Autodesk Inventor part; units mm, degrees
ref_plane "YZ Plane" through (0, 0, 0) normal (1, 0, 0) x (0, 1, 0)
ref_plane "XZ Plane" through (0, 0, 0) normal (0, 1, 0) x (-1, 0, 0)
ref_plane "XY Plane" through (0, 0, 0) normal (0, 0, 1) x (1, 0, 0)
sketch "スケッチ1" plane through (0, 0, 0) normal (0, 0, 1) x (1, 0, 0)
  line L0 (0, 0) -> (-57.5, 0)
  line L1 (-57.5, 0) -> (-57.5, 28)
  line L2 (-57.5, 28) -> (0, 28)
  line L3 (0, 28) -> (0, 0)
  line L4 (0, 14) -> (-110.5, 14)
  circle A0 centre (-110.5, 14) radius 53
  circle A1 centre (-110.5, 14) radius 23.5
  line L5 (0, 28) -> (-108.4685, 37.412)
  line L6 (0, 0) -> (-108.4685, -9.412)
  point P0 (-108.4685, -9.412)
  dimension "d3" = 47
  dimension "d0" = 28
  dimension "d1" = 57.5
  dimension "d2" = 106
extrude "押し出し1" add sketch "スケッチ1" along normal blind 3 contours L6 A0 L1 L0 | L0 L1 L4 L3 | L4 L1 L2 L3 | L6 A1 L4 A0 | A0 L5 L2 L1 | L4 A1 L5 A0 | A1
sketch "スケッチ2" plane through (0, 0, 3) normal (0, 0, 1) x (1, 0, 0)
  line L0 (0, 28) -> (-108.4685, 37.412)
  line L1 (0, 28) -> (-47.5, 28)
  line L2 (-47.5, 28) -> (-47.5, 0)
  line L3 (-47.5, 0) -> (0, 0)
  line L4 (0, 0) -> (0, 28)
  line L5 (-5, 28) -> (-5, 0)
  line L6 (-35, 28) -> (-35, 0)
  line L7 (0, 14) -> (-47.5, 14)
  point P0 (-35, 24)
  point P1 (-5, 24)
  point P2 (-35, 4)
  point P3 (-5, 4)
  dimension "d6" = 28
  dimension "d7" = 47.5
  dimension "d8" = 5
  dimension "d9" = 30
  dimension "d10" = 10
  dimension "d11" = 10
hole "穴1" at (-35, 24, 3) at (-5, 24, 3) at (-35, 4, 3) at (-5, 4, 3) direction (0, 0, -1) diameter 3.1 end through all
sketch "スケッチ3" plane through (0, 0, 3) normal (0, 0, 1) x (1, 0, 0)
  arc A0 (-108.4685, 37.412) -> (-108.4685, -9.412) centre (-110.5, 14) ccw
  circle A1 centre (-110.5, 14) radius 15.18
  circle A2 centre (-110.5, 14) radius 6
  line L0 (-110.5, 14) -> (-118.09, 27.1463)
  line L1 (-123.6463, 21.59) -> (-110.5, 14)
  line L2 (-110.5, 14) -> (-102.91, 27.1463)
  line L3 (-110.5, 14) -> (-110.5, 29.18)
  point P0 (0, 0)
  point P1 (-123.6463, 6.41)
  point P2 (-110.5, -1.18)
  point P3 (-97.3537, 6.41)
  point P4 (-97.3537, 21.59)
  point P5 (-110.5, 29.18)
  point P6 (-118.09, 0.8537)
  point P7 (-95.32, 14)
  dimension "d19" = 30.36
  dimension "d22" = 360
  dimension "d24" = 12
  dimension "d28" = 360
  dimension "d59" = 30
  dimension "d61" = 30
hole "穴2" at (-123.6463, 21.59, 3) at (-123.6463, 6.41, 3) at (-110.5, -1.18, 3) at (-97.3537, 6.41, 3) at (-97.3537, 21.59, 3) at (-110.5, 29.18, 3) at (-118.09, 27.1463, 3) at (-118.09, 0.8537, 3) at (-95.32, 14, 3) direction (0, 0, -1) diameter 4.1 end through all
sketch "スケッチ4" plane through (0, 0, 3) normal (0, 0, 1) x (1, 0, 0)
  arc A0 (-108.4685, 37.412) -> (-108.4685, -9.412) centre (-110.5, 14) ccw
  circle A1 centre (-110.5, 14) radius 10
  circle A2 centre (-110.5, 14) radius 23.5
  line L0 (-94.4636, -3.178) -> (0, 5.0188)
  line L1 (0, 0) -> (0, 28)
  line L2 (-108.4685, -9.412) -> (0, 0)
  line L3 (-94.4636, 31.178) -> (0, 22.9812)
  line L4 (0, 28) -> (-108.4685, 37.412)
  line L5 (-10, 23.8489) -> (-10, 4.1511)
  line L6 (-37.5, 26.2352) -> (-37.5, 1.7648)
  circle A3 centre (-35, 4) radius 1.55
  line L7 (-32.5, 25.8013) -> (-32.5, 2.1987)
  circle A4 centre (-35, 24) radius 1.55
  line L8 (-10, 23.8489) -> (-32.5, 2.1987)
  line L9 (-32.5, 5.6681) -> (-13.3073, 24.1359)
  line L10 (-28.537, 2.5426) -> (-10, 20.3795)
  line L11 (-62.5, 28.4045) -> (-62.5, -0.4045)
  line L12 (-57.5, 27.9706) -> (-57.5, 0.0294)
  line L13 (-57.5, 27.9706) -> (-37.5, 1.7648)
  line L14 (-57.5, 23.8499) -> (-40.4496, 1.5089)
  line L15 (-54.1321, 27.6784) -> (-37.5, 5.8856)
  line L16 (-94.4636, 31.178) -> (-94.4636, -3.178)
  line L17 (-91.4636, 30.9177) -> (-91.4636, -2.9177)
  line L18 (-62.5, 28.4045) -> (-91.4636, -2.9177)
  line L19 (-91.4636, 0.7646) -> (-65.6521, 28.678)
  line L20 (-87.7615, -2.5965) -> (-62.5, 24.7222)
  dimension "d37" = 20
  dimension "d38" = 5
  dimension "d39" = 5
  dimension "d40" = 10
  dimension "d41" = 2.5
  dimension "d42" = 2.5
  dimension "d43" = 2.5
  dimension "d44" = 2.5
  dimension "d45" = 5
  dimension "d46" = 20
  dimension "d47" = 2.5
  dimension "d48" = 2.5
  dimension "d49" = 3
  dimension "d50" = 2.5
  dimension "d51" = 2.5
extrude "押し出し2" cut sketch "スケッチ4" against normal blind 3 contours L17 L3 L19 A2 | A2 L19 L17 | L20 L11 L0 | L0 L10 L5 | L9 L7 L3 | L12 L14 L0 | L3 L6 L15 picked at (-90.6492, 17.3589)
fillet "フィレット1" radius 10 2 edges at (0, 28, 1.5) (0, 0, 1.5)
sketch "スケッチ5" plane through (0, 0, 3) normal (0, 0, 1) x (1, 0, 0)
  arc A0 (-108.4685, 37.412) -> (-108.4685, -9.412) centre (-110.5, 14) ccw
  circle A1 centre (-110.5, 14) radius 10
  point P0 (0, 0)
  dimension "d55" = 20
extrude "押し出し3" cut sketch "スケッチ5" against normal blind 3
properties part number "link1plate4" material "アルミニウム 6061"
The listing builds one solid part. Answer for the finished solid, in the listing's coordinates (mm). A direction names the side the tool comes from. Give positions to 0.01 mm unless a question says otherwise; leave off trailing zeros. Write each loop counter-clockwise with the first axis right and the second up, starting at its lowest first coordinate (ties: lowest second). Pieces come first, ordered by that corner, then holes.
1) A tool of negligible diameter and unlimited length cuts with its end or side. For faces 1 (the face through (-83, 9, 3)), 2 (the face through (-57.5, 12, 2)), from which of +Z, -Z, +X, -X, +Y, -Y can it reach the whole face along a straight path? Write none if from no direction.
2) Given P1, Ø2.5, axis at x = -118.09, y = 0.85, coming from the +Z side; P2, Ø1.5, axis at x = -103, z = 1.5, coming from the -Y side; P3, Ø1.5, axis at y = 26.5, z = 1, coming from the -X side, each flat-ended and moving along its own axis, determine where each tip first touches the part or whether it passes through.
3) For a pull along Y with two mould halves and no side action, classify faces 3 (the face through (-58.107, 33.042, 1.479)), 4 (the face through (-83, 9, 0)), 5 (the face through (-10, 12, 2)), 6 (the face through (-49.094, 12.836, 1.521)) as pulls with the +Y half, pulls with the -Y half, needs draft (parallel to the pull), parting line crosses it, or undercut.
4) Section A-A (x = -110.5) is taken. Write down the section's boundary in (y, z), and give its area (3 significant figures).
5) Section B-B (x = -26) is taken. Write down the section's boundary in (y, z).
6) Section C-C (y = 14) is taken. Count the separate pieces of the cut face and the enclosed holes in it, and give its area (3 significant figures).
7) Find the intervals of material crossed by L1, parallel to Y at x = -110.5, z = 1.6; L2, parallel to Y at x = -47, z = 0.85; L3, parallel to Y at x = -74.5, z = 0.6, in increasing order.
Response:
1. face 1: +Z, +X, -X, +Y, -Y
1. face 2: +Z, -Z
2. P1: passes through
2. P2: stops at y = -9
2. P3: stops at x = -130.85
3. face 3: pulls with the +Y half
3. face 4: needs draft
3. face 5: undercut
3. face 6: undercut
4. outline: (-9.5, 0) - (-3.23, 0) - (-3.23, 3) - (-9.5, 3) - close; (0.87, 0) - (4, 0) - (4, 3) - (0.87, 3) - close; (24, 0) - (27.13, 0) - (27.13, 3) - (24, 3) - close; (31.23, 0) - (37.5, 0) - (37.5, 3) - (31.23, 3) - close
4. area: 56.4 mm2
5. outline: (-2.26, 0) - (2.76, 0) - (2.76, 3) - (-2.26, 3) - close; (4.98, 0) - (11.92, 0) - (11.92, 3) - (4.98, 3) - close; (25.24, 0) - (30.26, 0) - (30.26, 3) - (25.24, 3) - close
6. separate pieces: 9
6. enclosed holes: 0
6. area: 176 mm2
7. L1: y = -9.5 to -3.23, 0.87 to 4, 24 to 27.13, 31.23 to 37.5
7. L2: y = -4.08 to 0.94, 10.09 to 18.33, 27.06 to 32.08
7. L3: y = -6.46 to -1.45, 11.74 to 19.11, 29.45 to 34.46
